Work out the finished part from the listing and answer in its coordinate system (mm). A direction names the side the tool comes from. Round coordinates to 2 decimals unless told otherwise and drop trailing zeros. Loops run counter-clockwise (first coordinate to the right, second up) from the corner with the lowest first, then second, coordinate; pieces in that order, holes last.
```python
from build123d import *

# Parameters (mm, degrees)
EXTRUDE_1_DEPTH     = 16.5
SKETCH_2_R          = 2.5
CUT_EXTRUDE_1_DEPTH = 16.5
SKETCH_3_W          = 10
SKETCH_3_H          = 16.5
CUT_EXTRUDE_2_DEPTH = 3
SKETCH_4_W          = 11.896315449
SKETCH_4_H          = 29.084641161
CUT_EXTRUDE_3_DEPTH = 48.945933091
SKETCH_5_R          = 2
CUT_EXTRUDE_4_DEPTH = 48.945933091
SKETCH_6_W          = 10
SKETCH_6_H          = 23
EXTRUDE_2_DEPTH     = 3
SKETCH_7_R          = 2.5
CUT_EXTRUDE_5_DEPTH = 3
EXTRUDE_START       = 3
SKETCH_8_R          = 2
SKETCH_8_W          = 6
SKETCH_8_H          = 26
EXTRUDE_3_DEPTH     = 3
SKETCH_9_R          = 2.5
CUT_EXTRUDE_6_DEPTH = 3
SKETCH_10_W         = 10
SKETCH_10_H         = 20
CUT_EXTRUDE_7_DEPTH = 10


with BuildPart() as part:
    # Sketch 1 → Extrude 1 (new body)
    with BuildSketch(Plane.XY):
        Polygon((0, 0), (26.75, 0), (26.75, -20), (36.75, -20), (36.75, -26), (20.75, -26), (20.75, -6), (0, -6), (-20.75, -6), (-20.75, -26), (-36.75, -26), (-36.75, -20), (-26.75, -20), (-26.75, 0), align=None)
    extrude(amount=EXTRUDE_1_DEPTH)

    # Sketch 2 → Cut-Extrude 1 (cut)
    with BuildSketch(Plane(origin=(0, -20, 0), x_dir=(1, 0, 0), z_dir=(0, 1, 0))):
        with Locations(Location((32.75, -8.25, 0), (0, 0, 270))):
            Circle(SKETCH_2_R)
    extrude(amount=-CUT_EXTRUDE_1_DEPTH, mode=Mode.SUBTRACT)

    # Sketch 3 → Cut-Extrude 2 (cut)
    with BuildSketch(Plane(origin=(0, -20, 0), x_dir=(1, 0, 0), z_dir=(0, 1, 0))):
        with Locations((31.75, -8.25)):
            Rectangle(SKETCH_3_W, SKETCH_3_H)
    extrude(amount=-CUT_EXTRUDE_2_DEPTH, mode=Mode.SUBTRACT)

    # Sketch 4 → Cut-Extrude 3 (cut, through all)
    with BuildSketch(Plane.XY.offset(16.5)):
        with Locations((-32.698157724, -14.542320581)):
            Rectangle(SKETCH_4_W, SKETCH_4_H)
    extrude(amount=-CUT_EXTRUDE_3_DEPTH, mode=Mode.SUBTRACT)

    # Sketch 5 → Cut-Extrude 4 (cut, through all)
    with BuildSketch(Plane(origin=(0, 0, 0), x_dir=(-1, 0, 0), z_dir=(0, 0, -1))):
        with Locations((-24.3, -11)):
            Circle(SKETCH_5_R)
        with Locations((-24.3, -21)):
            Circle(SKETCH_5_R)
        with Locations(Location((24.3, -21, 0), (0, 0, 180))):
            Circle(SKETCH_5_R)
        with Locations(Location((24.3, -11, 0), (0, 0, 180))):
            Circle(SKETCH_5_R)
    extrude(amount=-CUT_EXTRUDE_4_DEPTH, mode=Mode.SUBTRACT)

    # Sketch 6 → Extrude 2 (add)
    with BuildSketch(Plane(origin=(0, 0, 0), x_dir=(-1, 0, 0), z_dir=(0, 0, -1))):
        with Locations((-31.75, -34.5)):
            Rectangle(SKETCH_6_W, SKETCH_6_H)
    extrude(amount=EXTRUDE_2_DEPTH)

    # Sketch 7 → Cut-Extrude 5 (cut)
    with BuildSketch(Plane(origin=(0, 0, -3), x_dir=(-1, 0, 0), z_dir=(0, 0, -1))):
        with Locations((-31.75, -36)):
            Circle(SKETCH_7_R)
    extrude(amount=-CUT_EXTRUDE_5_DEPTH, mode=Mode.SUBTRACT)

    # Sketch 8 → Extrude 3 (add)
    # profile 1 of 2: a face of its own
    with BuildSketch(Plane(origin=(0, 0, 0), x_dir=(-1, 0, 0), z_dir=(0, 0, -1)).offset(EXTRUDE_START)):
        Polygon((26.75, 0), (20.75, 0), (20.75, -46), (26.75, -46), (30.75, -46), (30.75, -26), (26.75, -26), align=None)
        with Locations((24.3, -21)):
            Circle(SKETCH_8_R, mode=Mode.SUBTRACT)
        with Locations((24.3, -11)):
            Circle(SKETCH_8_R, mode=Mode.SUBTRACT)
    # profile 2 of 2: a face of its own
    with BuildSketch(Plane(origin=(0, 0, 0), x_dir=(-1, 0, 0), z_dir=(0, 0, -1)).offset(EXTRUDE_START)):
        with Locations((-23.75, -13)):
            Rectangle(SKETCH_8_W, SKETCH_8_H)
        with Locations((-24.3, -11)):
            Circle(SKETCH_8_R, mode=Mode.SUBTRACT)
        with Locations((-24.3, -21)):
            Circle(SKETCH_8_R, mode=Mode.SUBTRACT)
    extrude(amount=-EXTRUDE_3_DEPTH)

    # Sketch 9 → Cut-Extrude 6 (cut)
    with BuildSketch(Plane(origin=(0, 0, -3), x_dir=(-1, 0, 0), z_dir=(0, 0, -1))):
        with Locations((25.75, -36)):
            Circle(SKETCH_9_R)
    extrude(amount=-CUT_EXTRUDE_6_DEPTH, mode=Mode.SUBTRACT)

    # Sketch 10 → Cut-Extrude 7 (cut)
    with BuildSketch(Plane(origin=(0, 0, -3), x_dir=(-1, 0, 0), z_dir=(0, 0, -1))):
        with Locations((25.75, -36)):
            Rectangle(SKETCH_10_W, SKETCH_10_H)
    extrude(amount=-CUT_EXTRUDE_7_DEPTH, mode=Mode.SUBTRACT)


solid = part.part
```
1. Which of the six approach directions +Z, -Z, +X, -X, +Y, -Y give full straight-line access (tool end or side, diameter ignored) to faces 1 (the face through (33.59, -34.31, -1.52)), 2 (the face through (32, -23, 5)), 3 (the face through (0, -3, 0)), 4 (the face through (32.9, -33.6, 0)), 5 (the face through (26.75, -36, -1))?
Answer key:
face 1: +Z, -Z
face 2: +Z, -Z, +X, +Y
face 3: -Z, +Y, -Y
face 4: +Z, +X, -X, -Y
face 5: +Z, -Z, -X, -Y
2. Find section B-B (z = -0.75). Write down the section's boundary in (x, y).
Answer key:
outline: (-26.75, -26) - (-20.75, -26) - (-20.75, 0) - (-26.75, 0) - close; (20.75, -26) - (26.75, -26) - (26.75, -46) - (36.75, -46) - (36.75, -23) - (26.75, -23) - (26.75, 0) - (20.75, 0) - close; hole circle Ø4 at (-24.3, -21); hole circle Ø4 at (-24.3, -11); hole circle Ø4 at (24.3, -21); hole circle Ø4 at (24.3, -11); hole circle Ø5 at (31.75, -36)
3. Consider probe 1 along X at (y, z) = (-24.9, 8.25); probe 2 along Y at (x, z) = (24.3, 5.75); probe 3 along Y at (x, z) = (31.75, -1.25). Determine where each line is inside the solid, lowest interval first.
Answer key:
probe 1: x = -26.75 to -20.75, 20.75 to 30.25, 35.25 to 36.75
probe 2: y = -26 to -23, -19 to -13, -9 to 0
probe 3: y = -46 to -38.5, -33.5 to -23
4. Determine the mould class of faces 6 (the face through (36.75, -30.3, -0.4)), 7 (the face through (0, -6, 8)), 8 (the face through (29, -28, -3)) for opening direction X: +X half, -X half, draft (parallel to the pull), parting line (faces both ways), or undercut.
Answer key:
face 6: +X half
face 7: undercut
face 8: draft
5. Find section D-D (z = 3). Write down the section's boundary in (x, y).
Answer key:
outline: (-26.75, -26) - (-20.75, -26) - (-20.75, -6) - (20.75, -6) - (20.75, -26) - (36.75, -26) - (36.75, -23) - (26.75, -23) - (26.75, 0) - (-26.75, 0) - close; hole circle Ø4 at (-24.3, -21); hole circle Ø4 at (-24.3, -11); hole circle Ø4 at (24.3, -21); hole circle Ø4 at (24.3, -11)
6. Given pin 1 (2.5 mm diameter, centred on x = 24.3, y = -11, fed in from +Z); pin 2 (2 mm diameter, centred on x = 28.5, z = 1, fed in from +Y); pin 3 (6.5 mm diameter, centred on x = -22.5, z = 7.5, fed in from -Y); pin 4 (2.5 mm diameter, centred on y = -36, z = -1, fed in from -X), each flat-ended and moving along its own axis, determine where each tip first touches the part or whether it passes through.
Answer key:
pin 1: passes through
pin 2: stops at y = -23
pin 3: stops at y = -26
pin 4: stops at x = 26.75
7. Find section C-C (y = -14). Write down the section's boundary in (x, z).
Answer key:
outline: (-26.75, -3) - (-20.75, -3) - (-20.75, 16.5) - (-26.75, 16.5) - close; (20.75, -3) - (26.75, -3) - (26.75, 16.5) - (20.75, 16.5) - close
8. Find section A-A (x = 24.3). Write down the section's boundary in (y, z), then the cut area to 3 significant figures.
Answer key:
outline: (-26, -3) - (-23, -3) - (-23, 16.5) - (-26, 16.5) - close; (-19, -3) - (-13, -3) - (-13, 16.5) - (-19, 16.5) - close; (-9, -3) - (0, -3) - (0, 16.5) - (-9, 16.5) - close
area: 351 mm2
